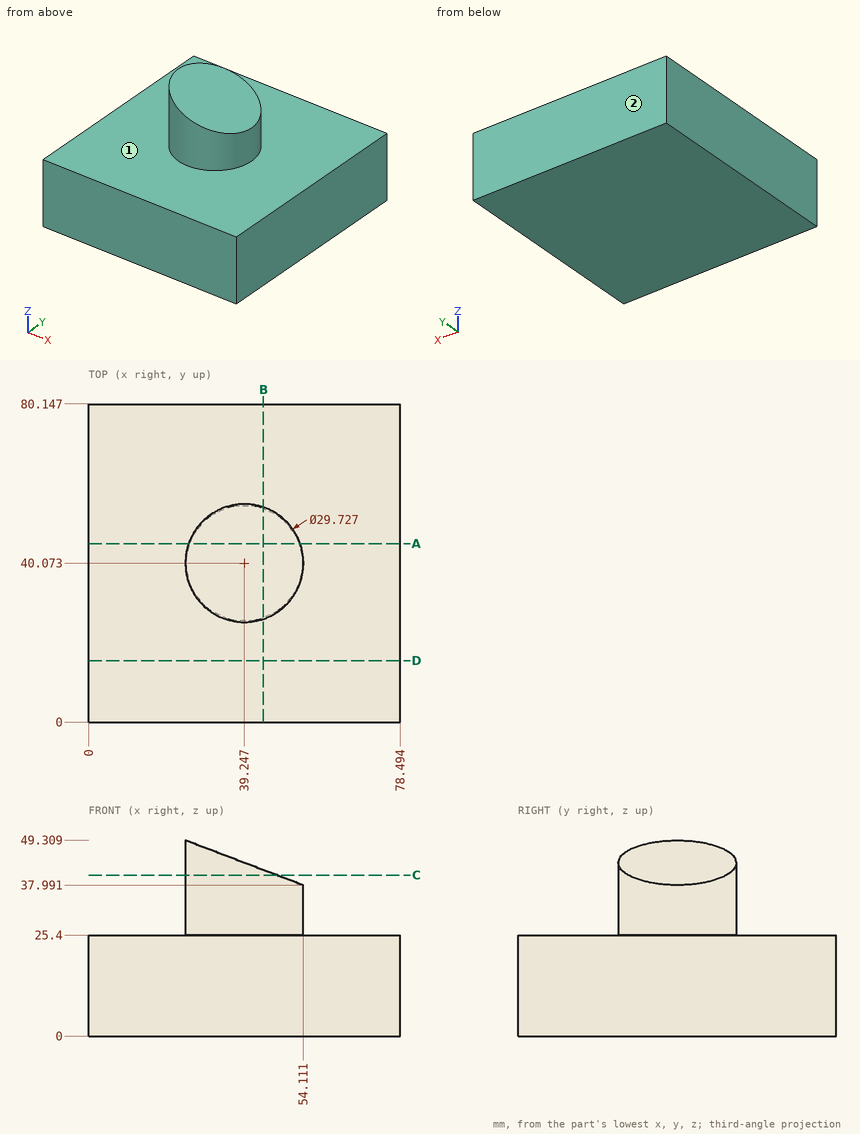
Geometry check sheet. Reference: drawing and pictorial views, mm from the part's lowest x, y, z. A direction names the side the tool comes from. Give positions to 0.01 mm unless a question says otherwise; leave off trailing zeros. Order: outer loops, then holes, each group sorted by start corner. A loop starts at its lowest first (then second) coordinate and runs counter-clockwise, first axis right, second up. Notation, with made-up numbers: (-21.5, 39) -> (-14.5, 39) arc R30 cw to (-14.5, 66) -> close; hole circle Ø6 at (9, 42). An arc over 180 degrees is marked (long way). Write each question's results on one line, items separated by ' | '. Start each with the question number.
(1) Sectioned sample at A-A (y = 45). Enter the section's corners in (x, z) (1 decimal).
(2) Sectioned sample at D-D (y = 15.5). Enter the section's corners in (x, z) (1 decimal).
(3) Scan lines: line 1 (Z direction, x = 11, y = 29); line 2 (Z direction, x = 30.5, y = 43); line 3 (X direction, y = 42, z = 27.5) (1 decimal). Record each from-to range of solid material in increasing order.
(4) Access from +Z, -Z, +X, -X, +Y, -Y to the whole of each face (thin tool, end or side, straight path). Record for the marked faces 1 and 2.
(5) Sectioned sample at B-B (x = 44). Enter the section's corners in (y, z).
(6) Gauge pin test, flat ends, axial feed: P1, Ø4, axis at x = 61.5, z = 14, coming from the -Y side; P2, Ø4, axis at x = 45.5, z = 41, coming from the -Y side; P3, Ø1, axis at y = 10.5, z = 26, coming from the +X side; P4, Ø3, axis at x = 10.5, y = 69.5, coming from the +Z side. Record the tip position at first contact, or that the pin passes through.
(7) Sectioned sample at C-C (z = 40.5). Enter the section's corners in (x, y) (1 decimal), plus the area to 3 significant figures.
Answer below:
1) outline: (0, 0) -> (78.5, 0) -> (78.5, 25.4) -> (53.3, 25.4) -> (53.3, 38.3) -> (25.2, 49) -> (25.2, 25.4) -> (0, 25.4) -> close
2) outline: (0, 0) -> (78.5, 0) -> (78.5, 25.4) -> (0, 25.4) -> close
3) line 1: 0 to 25.4 | line 2: 0 to 46.98 | line 3: 24.5 to 54
4) face 1: +Z | face 2: +Z, -Z, +X, -X, +Y
5) outline: (0, 0) -> (80.15, 0) -> (80.15, 25.4) -> (54.16, 25.4) -> (54.16, 41.84) -> (25.99, 41.84) -> (25.99, 25.4) -> (0, 25.4) -> close
6) P1: y = 0 | P2: y = 25.83 | P3: through | P4: z = 25.4
7) outline: (47.5, 27.7) -> (47.5, 52.4) arc R14.9 ccw (long way) to start | area: 580 mm2
